Read the model definition and answer for the solid it produces. Units are mm, in the model's axes. A direction names the side the tool comes from. Coordinates: 2 decimals unless noted, no trailing zeros. Write each loop counter-clockwise with the first axis right and the second up, starting at its lowest first coordinate (ties: lowest second). Pieces come first, ordered by that corner, then holes. Notation, with made-up numbers: M 39.5,-4.5 L 56.5,-4.5 A33 cw 56.5,31.5 Z; hole C 38.25,56 d6. An arc over 180 degrees is marked long. Write item = value, one per line.
from build123d import *

# Parameters (mm, degrees)
SKETCH_1_W      = 42
SKETCH_1_H      = 40
SKETCH_1_R      = 1.5
EXTRUDE_1_DEPTH = 3
SKETCH_3_W      = 40
SKETCH_3_H      = 49
SKETCH_3_R      = 11.5
SKETCH_3_R_2    = 1.5
EXTRUDE_2_DEPTH = 3
FILLET_1_R      = 5
FILLET_2_R      = 5


with BuildPart() as part:
    # 草图1 → 凸台-拉伸1 (new body)
    with BuildSketch(Plane(origin=(0, 0, 0), x_dir=(1, 0, 0), z_dir=(0, 1, 0))):
        Rectangle(SKETCH_1_W, SKETCH_1_H)
        with Locations(Location((-12, 15, 0), (0, 0, 270))):
            Circle(SKETCH_1_R, mode=Mode.SUBTRACT)
        with Locations(Location((-12, -15, 0), (0, 0, 90))):
            Circle(SKETCH_1_R, mode=Mode.SUBTRACT)
        with Locations(Location((12, -15, 0), (0, 0, 270))):
            Circle(SKETCH_1_R, mode=Mode.SUBTRACT)
        with Locations(Location((12, 15, 0), (0, 0, 90))):
            Circle(SKETCH_1_R, mode=Mode.SUBTRACT)
    extrude(amount=EXTRUDE_1_DEPTH)

    # 草图3 → 凸台-拉伸2 (add)
    with BuildSketch(Plane.ZY.offset(21)):
        with Locations((0, 27.5)):
            Rectangle(SKETCH_3_W, SKETCH_3_H)
        with Locations((0, 31)):
            Circle(SKETCH_3_R, mode=Mode.SUBTRACT)
        with Locations((-15.5, 46.5)):
            Circle(SKETCH_3_R_2, mode=Mode.SUBTRACT)
        with Locations((-15.5, 15.5)):
            Circle(SKETCH_3_R_2, mode=Mode.SUBTRACT)
        with Locations(Location((15.5, 15.5, 0), (0, 0, 180))):
            Circle(SKETCH_3_R_2, mode=Mode.SUBTRACT)
        with Locations(Location((15.5, 46.5, 0), (0, 0, 180))):
            Circle(SKETCH_3_R_2, mode=Mode.SUBTRACT)
    extrude(amount=-EXTRUDE_2_DEPTH)

    # 圆角1
    fillet_1_edges = [part.edges().sort_by_distance(p)[0] for p in [
        (-19.5, 52, -20),
        (-19.5, 52, 20),
    ]]
    fillet(fillet_1_edges, radius=FILLET_1_R)

    # 圆角2
    fillet_2_edges = [part.edges().sort_by_distance(p)[0] for p in [
        (21, 1.5, 20),
        (21, 1.5, -20),
    ]]
    fillet(fillet_2_edges, radius=FILLET_2_R)


solid = part.part
Item 1: Which of the six approach directions +Z, -Z, +X, -X, +Y, -Y give full straight-line access (tool end or side, diameter ignored) to faces 1 (the face through (1, 3, 0)), 2 (the face through (0, 0, 0))?
Worked answers:
face_1 = +Z, -Z, +X, +Y
face_2 = +Z, -Z, +X, -X, -Y
Item 2: For a pull along X with two mould halves and no side action, classify faces 3 (the face through (-21, 21, -9)), 4 (the face through (-19.52, 15.43, 17)), 5 (the face through (12.07, 1.48, 13.5)) as released by +X, released by -X, zero draft, split by the parting line, or undercut.
Worked answers:
face_3 = released by -X
face_4 = zero draft
face_5 = undercut
Item 3: Find section A-A (z = 0). Determine the outline of the cut face in (x, y), and give its area (3 significant figures).
Worked answers:
outline = M -21,0 L 21,0 L 21,3 L -18,3 L -18,19.5 L -21,19.5 Z; M -21,42.5 L -18,42.5 L -18,52 L -21,52 Z
area = 204 mm²
Item 4: Find section D-D (y = 15.5). Determine the outline of the cut face in (x, z).
Worked answers:
outline = M -21,-20 L -18,-20 L -18,-17 L -21,-17 Z; M -21,-14 L -18,-14 L -18,14 L -21,14 Z; M -21,17 L -18,17 L -18,20 L -21,20 Z
Item 5: Consider line 1 along X through (y, z) = (1, -15); line 2 along Y through (x, z) = (-8.5, -1.5); line 3 along X through (y, z) = (19, -12.5). Determine where each line is inside the solid, lowest interval first. Write a range as from..to.
Worked answers:
line_1 = -21..-13.5, -10.5..10.5, 13.5..21
line_2 = 0..3
line_3 = -21..-18
Item 6: Find section B-B (y = 31). Determine the outline of the cut face in (x, z).
Worked answers:
outline = M -21,-20 L -18,-20 L -18,-11.5 L -21,-11.5 Z; M -21,11.5 L -18,11.5 L -18,20 L -21,20 Z
Item 7: Find section C-C (x = 12). Determine the outline of the cut face in (y, z).
Worked answers:
outline = M 0,-20 L 3,-20 L 3,-16.5 L 0,-16.5 Z; M 0,-13.5 L 3,-13.5 L 3,13.5 L 0,13.5 Z; M 0,16.5 L 3,16.5 L 3,20 L 0,20 Z
Item 8: Flat-ended cylindrical pins translate along their axes: pin 1 (2.5 mm diameter, centred on x = 12, z = -15, fed in from +Y); pin 2 (3.5 mm diameter, centred on x = 12, z = 15, fed in from +Y); pin 3 (5 mm diameter, centred on y = 9, z = -2, fed in from +X). Find the tip coordinate at first contact, or state that the pin passes through.
Worked answers:
pin_1 = through
pin_2 = 3
pin_3 = -18
